For this review, take the finished solid that the model builds, in its own axes (mm). Round coordinates to 2 decimals unless told otherwise and drop trailing zeros. Write each question's results on one line, items separated by ' | '.
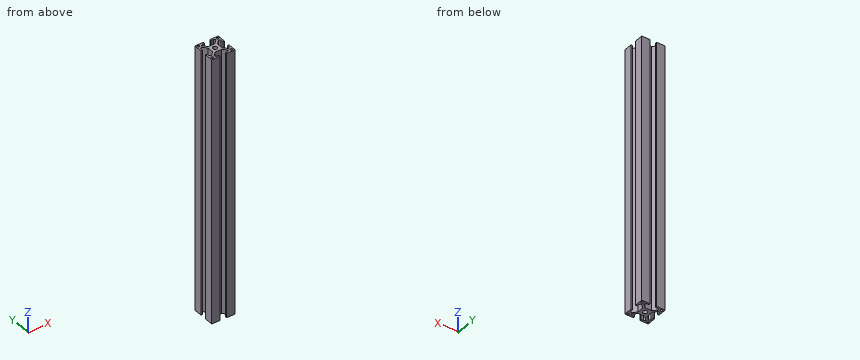
Autodesk Inventor part; units mm, degrees
ref_plane "YZ Plane" through (0, 0, 0) normal (1, 0, 0) x (0, 1, 0)
ref_plane "XZ Plane" through (0, 0, 0) normal (0, 1, 0) x (-1, 0, 0)
ref_plane "XY Plane" through (0, 0, 0) normal (0, 0, 1) x (1, 0, 0)
sketch "Sketch1" plane through (0, 0, 0) normal (0, 0, 1) x (1, 0, 0)
  line L0 (0, 0) -> (8, 0)
  line L1 (8, 0) -> (8, -1.5)
  line L2 (8, -1.5) -> (5.5711, -1.5)
  line L3 (0, -1.5) -> (0, 0)
  line L4 (0, 0) -> (5, 0) construction
  line L5 (4.2426, -2.8284) -> (5.5711, -1.5)
  line L6 (6.5, -14.0858) -> (6.5, -7.9142)
  line L7 (7.9142, -6.5) -> (15.5, -6.5)
  line L8 (0, -8) -> (1.5, -8)
  line L9 (1.5, -8) -> (1.5, -5.5711)
  line L10 (11, -11) -> (10.2929, -10.2929) construction
  line L11 (11, -11) -> (10.2929, -11.7071) construction
  line L12 (0, 0) -> (8, 0)
  line L13 (5.5711, -1.5) -> (4.2426, -2.8284)
  line L14 (2.8284, -4.2426) -> (1.5, -5.5711)
  line L15 (7.9142, -6.5) -> (4.2426, -2.8284)
  line L16 (6.5, -7.9142) -> (2.8284, -4.2426)
  circle A0 centre (11, -11) radius 2
  line L17 (11, -11) -> (16.6687, -11) construction
  line L18 (11, -16.9105) -> (11, -11) construction
  line L19 (22, 0) -> (14, 0)
  line L20 (14, 0) -> (14, -1.5)
  line L21 (14, -1.5) -> (16.4289, -1.5)
  line L22 (22, -1.5) -> (22, 0)
  line L23 (22, 0) -> (17, 0)
  line L24 (17.7574, -2.8284) -> (16.4289, -1.5)
  line L25 (15.5, -15.5) -> (15.5, -7.9142)
  line L26 (15.5, -6.5) -> (7.9142, -6.5)
  line L27 (22, -8) -> (20.5, -8)
  line L28 (20.5, -8) -> (20.5, -5.5711)
  line L29 (11, -11) -> (11.7071, -10.2929) construction
  line L30 (11, -11) -> (11.7071, -11.7071) construction
  line L31 (22, 0) -> (14, 0)
  line L32 (16.4289, -1.5) -> (17.7574, -2.8284)
  line L33 (19.1716, -4.2426) -> (20.5, -5.5711)
  line L34 (14.0858, -6.5) -> (17.7574, -2.8284)
  line L35 (15.5, -7.9142) -> (19.1716, -4.2426)
  circle A1 centre (11, -11) radius 2
  line L36 (0, -22) -> (8, -22)
  line L37 (8, -22) -> (8, -20.5)
  line L38 (8, -20.5) -> (5.5711, -20.5)
  line L39 (0, -20.5) -> (0, -22)
  line L40 (0, -22) -> (5, -22) construction
  line L41 (4.2426, -19.1716) -> (5.5711, -20.5)
  line L42 (6.5, -7.9142) -> (6.5, -14.0858)
  line L43 (6.5, -15.5) -> (14.0858, -15.5)
  line L44 (0, -14) -> (1.5, -14)
  line L45 (1.5, -14) -> (1.5, -16.4289)
  line L46 (11, -11) -> (10.2929, -11.7071) construction
  line L47 (11, -11) -> (10.2929, -10.2929) construction
  line L48 (0, -22) -> (8, -22)
  line L49 (5.5711, -20.5) -> (4.2426, -19.1716)
  line L50 (2.8284, -17.7574) -> (1.5, -16.4289)
  line L51 (7.9142, -15.5) -> (4.2426, -19.1716)
  line L52 (6.5, -14.0858) -> (2.8284, -17.7574)
  circle A2 centre (11, -11) radius 2
  line L53 (22, -22) -> (14, -22)
  line L54 (14, -22) -> (14, -20.5)
  line L55 (14, -20.5) -> (16.4289, -20.5)
  line L56 (22, -20.5) -> (22, -22)
  line L57 (22, -22) -> (17, -22)
  line L58 (17.7574, -19.1716) -> (16.4289, -20.5)
  line L59 (20.5, -14) -> (20.5, -16.4289)
  line L60 (15.5, -14.0858) -> (19.1716, -17.7574)
  line L61 (19.1716, -17.7574) -> (20.5, -16.4289)
  line L62 (14.0858, -15.5) -> (17.7574, -19.1716)
  line L63 (16.4289, -20.5) -> (17.7574, -19.1716)
  line L64 (22, -22) -> (14, -22)
  line L65 (22, -14) -> (20.5, -14)
  line L66 (11, -11) -> (11.7071, -11.7071) construction
  line L67 (11, -11) -> (11.7071, -10.2929) construction
  line L68 (14.0858, -15.5) -> (6.5, -15.5)
  line L69 (15.5, -7.9142) -> (15.5, -15.5)
  circle A3 centre (11, -11) radius 2
  line L70 (22, -14) -> (22, -20.5)
  line L71 (22, -1.5) -> (22, -8)
  line L72 (8, 0) -> (0, 0) construction
  line L73 (0, 0) -> (0, -8) construction
  line L74 (9.5858, -11) -> (9.0681, -11.5176)
  line L75 (6.5, -14.0858) -> (2.8284, -17.7574)
  line L76 (0, -22) -> (0, -14)
  line L77 (0, -8) -> (0, 0)
  line L78 (0, 0) -> (2, 0) construction
  line L79 (2, 0) -> (2, -2) construction
  circle A4 centre (2, -2) radius 1
  circle A5 centre (20, -2) radius 1
  circle A6 centre (2, -20) radius 1
  circle A7 centre (20, -20) radius 1
  point P0 (3.5355, -3.5355)
  point P1 (0, -7.0711)
  point P2 (6.5, -6.5)
  point P3 (6.5, -15.5)
  point P4 (1.5, 0)
  point P5 (10.2929, -10.2929)
  point P6 (18.4645, -3.5355)
  point P7 (22, -7.0711)
  point P8 (6.5, -6.5)
  point P9 (20.5, 0)
  point P10 (11.7071, -10.2929)
  point P11 (12.4142, -11)
  point P12 (3.5355, -18.4645)
  point P13 (0, -14.9289)
  point P14 (6.5, -6.5)
  point P15 (1.5, -22)
  point P16 (10.2929, -11.7071)
  point P17 (18.4645, -18.4645)
  point P18 (20.5, -22)
  point P19 (22, -14.9289)
  point P20 (15.5, -6.5)
  point P21 (11.7071, -11.7071)
  dimension "d2" = 8
  dimension "d3" = 1.5
  dimension "d4" = 5
  dimension "d10" = 9
  dimension "d11" = 9
  dimension "d14" = 4
  dimension "d15" = 2
  dimension "d16" = 2
  dimension "d17" = 2
extrude "Extrusion1" add sketch "Sketch1" along normal blind 250
properties part number "extrusion_250"
1. For pin 1 (1.2 mm diameter, centred on x = 20, y = -20, fed in from +Z); pin 2 (3 mm diameter, centred on x = 11, z = 71, fed in from +Y); pin 3 (1.9 mm diameter, centred on y = -11, z = 95, fed in from -X), all flat-tipped, find the tip position at first contact; note any pin that passes through.
Values found:
pin 1: passes through | pin 2: stops at y = -6.5 | pin 3: stops at x = 6.5
2. To check wall thickness, follow probe 1 along Y at (x, z) = (11, 131.5); probe 2 along Y at (x, z) = (19.25, 61.5); probe 3 along Y at (x, z) = (2, 186). State the ranges of each line that lie inside material, in increasing order.
Values found:
probe 1: y = -15.5 to -13, -9 to -6.5 | probe 2: y = -22 to -20.66, -19.34 to -17.68, -4.32 to -2.66, -1.34 to 0 | probe 3: y = -22 to -21, -19 to -16.93, -5.07 to -3, -1 to 0
3. Consider section A-A (z = 203). Give the number of separate pieces and of enclosed holes in the cut face, plus the area to 3 significant figures.
Values found:
separate pieces: 1 | enclosed holes: 5 | area: 214 mm2
